from build123d import *

# Parameters (mm, degrees)
F0_R     = 10
F1_DEPTH = 3


with BuildPart() as f1:
    # F0 (on Front) → F1 (new body)
    with BuildSketch(Plane.XZ):
        with BuildLine():
            Line((-3.915787, 72.004935), (-11.747279, 65.150152))
            ThreePointArc((-11.747279, 65.150152), (-15.061523, 62.859987), (-17.66665, 65.932834))
            Line((-17.66665, 65.932834), (-17.469185, 71.929583))
            Line((-17.469185, 71.929583), (-22.418608, 68.537946))
            Line((-22.418608, 68.537946), (-28.209101, 59.889795))
            ThreePointArc((-28.209101, 59.889795), (-30.817676, 56.819876), (-34.129346, 59.113761))
            Line((-34.129346, 59.113761), (-35.490683, 64.957285))
            Line((-35.490683, 64.957285), (-39.393639, 60.400209))
            Line((-39.393639, 60.400209), (-42.748518, 50.548047))
            ThreePointArc((-42.748518, 50.548047), (-44.473655, 46.907584), (-48.266184, 48.266184))
            Line((-48.266184, 48.266184), (-51.093549, 53.558254))
            Line((-51.093549, 53.558254), (-53.684057, 48.146298))
            Line((-53.684057, 48.146298), (-54.374695, 37.761533))
            ThreePointArc((-54.374695, 37.761533), (-55.098828, 33.798618), (-59.113761, 34.129346))
            Line((-59.113761, 34.129346), (-63.214475, 38.509317))
            Line((-63.214475, 38.509317), (-64.315996, 32.611296))
            Line((-64.315996, 32.611296), (-62.295326, 22.401634))
            ThreePointArc((-62.295326, 22.401634), (-61.969107, 18.386332), (-65.932834, 17.66665))
            Line((-65.932834, 17.66665), (-71.027439, 20.836034))
            Line((-71.027439, 20.836034), (-70.564907, 14.853889))
            Line((-70.564907, 14.853889), (-65.970634, 5.5151))
            ThreePointArc((-65.970634, 5.5151), (-64.616294, 1.721047), (-68.258692, 0))
            Line((-68.258692, 0), (-74, 1.742809))
            Line((-74, 1.742809), (-72.004935, -3.915787))
            Line((-72.004935, -3.915787), (-65.150152, -11.747279))
            ThreePointArc((-65.150152, -11.747279), (-62.859987, -15.061523), (-65.932834, -17.66665))
            Line((-65.932834, -17.66665), (-71.929583, -17.469185))
            Line((-71.929583, -17.469185), (-68.537946, -22.418608))
            Line((-68.537946, -22.418608), (-59.889795, -28.209101))
            ThreePointArc((-59.889795, -28.209101), (-56.819876, -30.817676), (-59.113761, -34.129346))
            Line((-59.113761, -34.129346), (-64.957285, -35.490683))
            Line((-64.957285, -35.490683), (-60.400209, -39.393639))
            Line((-60.400209, -39.393639), (-50.548047, -42.748518))
            ThreePointArc((-50.548047, -42.748518), (-46.907584, -44.473655), (-48.266184, -48.266184))
            Line((-48.266184, -48.266184), (-53.558254, -51.093549))
            Line((-53.558254, -51.093549), (-48.146298, -53.684057))
            Line((-48.146298, -53.684057), (-37.761533, -54.374695))
            ThreePointArc((-37.761533, -54.374695), (-33.798618, -55.098828), (-34.129346, -59.113761))
            Line((-34.129346, -59.113761), (-38.509317, -63.214475))
            Line((-38.509317, -63.214475), (-32.611296, -64.315996))
            Line((-32.611296, -64.315996), (-22.401634, -62.295326))
            ThreePointArc((-22.401634, -62.295326), (-18.386332, -61.969107), (-17.66665, -65.932834))
            Line((-17.66665, -65.932834), (-20.836034, -71.027439))
            Line((-20.836034, -71.027439), (-14.853889, -70.564907))
            Line((-14.853889, -70.564907), (-5.5151, -65.970634))
            ThreePointArc((-5.5151, -65.970634), (-1.721047, -64.616294), (0, -68.258692))
            Line((0, -68.258692), (-1.742809, -74))
            Line((-1.742809, -74), (3.915787, -72.004935))
            Line((3.915787, -72.004935), (11.747279, -65.150152))
            ThreePointArc((11.747279, -65.150152), (15.061523, -62.859987), (17.66665, -65.932834))
            Line((17.66665, -65.932834), (17.469185, -71.929583))
            Line((17.469185, -71.929583), (22.418608, -68.537946))
            Line((22.418608, -68.537946), (28.209101, -59.889795))
            ThreePointArc((28.209101, -59.889795), (30.817676, -56.819876), (34.129346, -59.113761))
            Line((34.129346, -59.113761), (35.490683, -64.957285))
            Line((35.490683, -64.957285), (39.393639, -60.400209))
            Line((39.393639, -60.400209), (42.748518, -50.548047))
            ThreePointArc((42.748518, -50.548047), (44.473655, -46.907584), (48.266184, -48.266184))
            Line((48.266184, -48.266184), (51.093549, -53.558254))
            Line((51.093549, -53.558254), (53.684057, -48.146298))
            Line((53.684057, -48.146298), (54.374695, -37.761533))
            ThreePointArc((54.374695, -37.761533), (55.098828, -33.798618), (59.113761, -34.129346))
            Line((59.113761, -34.129346), (63.214475, -38.509317))
            Line((63.214475, -38.509317), (64.315996, -32.611296))
            Line((64.315996, -32.611296), (62.295326, -22.401634))
            ThreePointArc((62.295326, -22.401634), (61.969107, -18.386332), (65.932834, -17.66665))
            Line((65.932834, -17.66665), (71.027439, -20.836034))
            Line((71.027439, -20.836034), (70.564907, -14.853889))
            Line((70.564907, -14.853889), (65.970634, -5.5151))
            ThreePointArc((65.970634, -5.5151), (64.616294, -1.721047), (68.258692, 0))
            Line((68.258692, 0), (74, -1.742809))
            Line((74, -1.742809), (72.004935, 3.915787))
            Line((72.004935, 3.915787), (65.150152, 11.747279))
            ThreePointArc((65.150152, 11.747279), (62.859987, 15.061523), (65.932834, 17.66665))
            Line((65.932834, 17.66665), (71.929583, 17.469185))
            Line((71.929583, 17.469185), (68.537946, 22.418608))
            Line((68.537946, 22.418608), (59.889795, 28.209101))
            ThreePointArc((59.889795, 28.209101), (56.819876, 30.817676), (59.113761, 34.129346))
            Line((59.113761, 34.129346), (64.957285, 35.490683))
            Line((64.957285, 35.490683), (60.400209, 39.393639))
            Line((60.400209, 39.393639), (50.548047, 42.748518))
            ThreePointArc((50.548047, 42.748518), (46.907584, 44.473655), (48.266184, 48.266184))
            Line((48.266184, 48.266184), (53.558254, 51.093549))
            Line((53.558254, 51.093549), (48.146298, 53.684057))
            Line((48.146298, 53.684057), (37.761533, 54.374695))
            ThreePointArc((37.761533, 54.374695), (33.798618, 55.098828), (34.129346, 59.113761))
            Line((34.129346, 59.113761), (38.509317, 63.214475))
            Line((38.509317, 63.214475), (32.611296, 64.315996))
            Line((32.611296, 64.315996), (22.401634, 62.295326))
            ThreePointArc((22.401634, 62.295326), (18.386332, 61.969107), (17.66665, 65.932834))
            Line((17.66665, 65.932834), (20.836034, 71.027439))
            Line((20.836034, 71.027439), (14.853889, 70.564907))
            Line((14.853889, 70.564907), (5.5151, 65.970634))
            ThreePointArc((5.5151, 65.970634), (1.721047, 64.616294), (0, 68.258692))
            Line((0, 68.258692), (1.742809, 74))
            Line((1.742809, 74), (-3.915787, 72.004935))
        make_face()
        Circle(F0_R, mode=Mode.SUBTRACT)
    extrude(amount=F1_DEPTH)


solid = f1.part
Design review of the part built by this model. Coordinates are the model's own, in mm. A direction names the side the tool comes from. Round coordinates to 2 decimals unless told otherwise and drop trailing zeros. Write each loop counter-clockwise with the first axis right and the second up, starting at its lowest first coordinate (ties: lowest second). Pieces come first, ordered by that corner, then holes. Notation, with made-up numbers: (-1.5, 17) - (10.5, 17) arc R24 cw to (10.5, 51) - close; hole circle Ø4 at (-1, 70). An arc over 180 degrees is marked (long way). Return JSON: item names as keys, results as strings. Group by question number.
Item 1: We need section A-A on z = -45. Write out the cut boundary in (x, y), and give its area (3 significant figures).
Item 2: For probe 1 along X at (y, z) = (-1, 67); probe 2 along X at (y, z) = (-2.25, 18.5); probe 3 along X at (y, z) = (-2.7, 18), list the stretches that pass through material, from the lowest coordinate up. Write a range as [from, to].
Item 3: Insertion check: P1, Ø4, axis at x = -58, z = -8.5, coming from the +Y side. The pin has a flat end and moves straight along its axis. Give the tip position at first contact, or say it passes through.
Item 4: Machinability: for faces 4 (the face through (-68.626, -1.479, -7.777)), 5 (the face through (-62.711, -1.479, -37.415)), 6 (the face through (64.274, -1.479, 25.273)), 7 (the face through (61.135, -1.479, -36.289)), 8 (the face through (10.25, -1.48, 68.3)), which of the approach directions +Z, -Z, +X, -X, +Y, -Y give a long, thin tool a straight path to every point of the face, cutting with its end or side? Answer none if there is none.
Item 5: The part is to be moulded in two halves that separate along X. For faces 1 (the face through (19.2, -1.5, 68.4)), 2 (the face through (-68.3, -1.48, 10.25)), 3 (the face through (25.273, -1.479, -64.274)), say which applies: pulls with the +X half, pulls with the -X half, needs draft (parallel to the pull), parting line crosses it, or undercut.
Item 6: We need section B-B on z = -24.5. Write out the cut boundary in (x, y).
Model answer:
{
 "1": {"outline": "(-46.74, -3) - (53.89, -3) - (53.89, 0) - (-46.74, 0) - close", "area": "302 mm²"},
 "2": {"probe 1": "x = [-23.45, -17.63], [-9.63, -0.1], [7.61, 18.33]", "probe 2": "x = [-70.85, -67.27], [-61.89, 71.22]", "probe 3": "x = [-70.81, -66.47], [-62.32, 71.57]"},
 "3": {"P1": "stops at y = 0"},
 "4": {"face 4": "-X, +Y, -Y", "face 5": "-Z, -X, +Y, -Y", "face 6": "+X, +Y, -Y", "face 7": "-Z, +Y, -Y", "face 8": "+Z, +Y, -Y"},
 "5": {"face 1": "pulls with the +X half", "face 2": "pulls with the -X half", "face 3": "undercut"},
 "6": {"outline": "(-65.43, -3) - (62.71, -3) - (62.71, 0) - (-65.43, 0) - close"}
}
